Source: CAD feature listing. Evaluate the final solid. Frame: model axes, mm. A direction names the side the tool comes from. Coordinates: 2 decimals unless noted, no trailing zeros. Write each loop counter-clockwise with the first axis right and the second up, starting at its lowest first coordinate (ties: lowest second). Pieces come first, ordered by that corner, then holes. Notation, with made-up numbers: (67.5, 17) - (86.5, 17) arc R17 ccw to (86.5, 43) - close; hole circle Ø4 at (52.5, 86.5). An arc over 180 degrees is marked (long way). One line per question, with ' | ' between items. Start each with the question number.
Q1. Draft query along Y for faces 1 (the face through (78, 16.18, 35)), 2 (the face through (13.92, -8.8, 12.88)), 3 (the face through (80, -19.05, 13)). Return one class per face: +Y half, -Y half, draft (parallel to the pull), parting line (faces both ways), or undercut.
Q2. Cut plane B-B, the plane y = -13. Return loops of the section in (x, z) (3 decimals).
Q3. Access query for faces 4 (the face through (49.098, 0, -2)), 5 (the face through (79, 16.18, -2)), 6 (the face through (49.098, 0, 35)). Directions: +Z, -Z, +X, -X, +Y, -Y. A direction counts if a zero-diameter tool reaches every point of the face in a straight line with its end or side. Return the directions, or none.
Q4. Contact query for flat-ended pins moving along their axis: P1, Ø12, axis at x = 120, z = 35.5, coming from the -Y side; P2, Ø3.5, axis at y = 0.5, z = -3, coming from the +X side; P3, Ø6, axis at y = -7.5, z = 30.5, coming from the -X side; P4, Ø3.5, axis at x = 77.5, z = -3, coming from the +Y side. Output: stop coordinate, or through.
Q5. Cut plane D-D, the plane x = 65.5. Return loops of the section in (y, z).
Q6. Cut plane A-A, the plane x = 25.4. Return loops of the section in (y, z).
Q7. Line query: line 1 (Y direction, x = 25.4, z = 14.5); line 2 (Z direction, x = 7, y = 6); line 3 (X direction, y = 0, z = 33). Output: solid intervals per line, ascending.
Q8. Cut plane C-C, the plane z = 22. Return loops of the section in (x, y) (3 decimals), plus the area to 3 significant figures.
```python
from build123d import *

# Parameters (mm, degrees)
SKETCH1_W           = 161.925
SKETCH1_H           = 38.1
BOSS_EXTRUDE1_DEPTH = 25.4
SKETCH3_W           = 59.182
SKETCH3_H           = 32.3596
BOSS_EXTRUDE3_DEPTH = 19.7866
SKETCH4_W           = 59.182
SKETCH4_H           = 32.3596
BOSS_EXTRUDE4_DEPTH = 4.2926
SKETCH6_R           = 14.4653
CUT_EXTRUDE1_DEPTH  = 30.6926


with BuildPart() as part:
    # Sketch1 → Boss-Extrude1 (new body)
    with BuildSketch(Plane.XY):
        with Locations((80.9625, 0)):
            Rectangle(SKETCH1_W, SKETCH1_H)
    extrude(amount=BOSS_EXTRUDE1_DEPTH)

    # Sketch3 → Boss-Extrude3 (add)
    with BuildSketch(Plane.XY.offset(25.4)):
        with Locations((78.6892, 0)):
            Rectangle(SKETCH3_W, SKETCH3_H)
    extrude(amount=BOSS_EXTRUDE3_DEPTH)

    # Sketch4 → Boss-Extrude4 (add)
    with BuildSketch(Plane(origin=(0, 0, 0), x_dir=(-1, 0, 0), z_dir=(0, 0, -1))):
        with Locations((-78.6892, 0)):
            Rectangle(SKETCH4_W, SKETCH4_H)
    extrude(amount=BOSS_EXTRUDE4_DEPTH)

    # Sketch6 → Cut-Extrude1 (cut, through all)
    with BuildSketch(Plane.XY.offset(25.4)):
        with Locations((25.4, 0)):
            Circle(SKETCH6_R)
    extrude(amount=-CUT_EXTRUDE1_DEPTH, mode=Mode.SUBTRACT)


solid = part.part
```
Reply:
1) face 1: +Y half | face 2: undercut | face 3: -Y half
2) outline: (0, 0) - (19.056, 0) - (19.056, 25.4) - (0, 25.4) - close; (31.744, 0) - (49.098, 0) - (49.098, -4.293) - (108.28, -4.293) - (108.28, 0) - (161.925, 0) - (161.925, 25.4) - (108.28, 25.4) - (108.28, 45.187) - (49.098, 45.187) - (49.098, 25.4) - (31.744, 25.4) - close
3) face 4: -Z, -X, +Y, -Y | face 5: -Z, +X, -X, +Y | face 6: +Z, -X, +Y, -Y
4) P1: passes through | P2: stops at x = 108.28 | P3: stops at x = 49.1 | P4: stops at y = 16.18
5) outline: (-19.05, 0) - (-16.18, 0) - (-16.18, -4.29) - (16.18, -4.29) - (16.18, 0) - (19.05, 0) - (19.05, 25.4) - (16.18, 25.4) - (16.18, 45.19) - (-16.18, 45.19) - (-16.18, 25.4) - (-19.05, 25.4) - close
6) outline: (-19.05, 0) - (-14.47, 0) - (-14.47, 25.4) - (-19.05, 25.4) - close; (14.47, 0) - (19.05, 0) - (19.05, 25.4) - (14.47, 25.4) - close
7) line 1: y = -19.05 to -14.47, 14.47 to 19.05 | line 2: z = 0 to 25.4 | line 3: x = 49.1 to 108.28
8) outline: (0, -19.05) - (161.925, -19.05) - (161.925, 19.05) - (0, 19.05) - close; hole circle Ø28.931 at (25.4, 0) | area: 5,510 mm^2
